```python
from build123d import *

# Parameters (mm, degrees)
F0_W      = 807.212
F0_H      = 403.86
F1_DEPTH  = 250.444
F2_R      = 60.325
F3_DEPTH  = 49.276
F4_T      = -25.4
F5_R      = 65.0773908114
F6_DEPTH  = 222.25
F7_R      = 62.8893110404
F8_DEPTH  = 222.25
F9_R      = 59.4615536077
F10_DEPTH = 222.25
F11_T     = -7.62


with BuildPart() as f1:
    # F0 (on Front) → F1 (new body)
    with BuildSketch(Plane.XZ):
        with Locations((41.8836543641, 201.93)):
            Rectangle(F0_W, F0_H)
    extrude(amount=F1_DEPTH)

    # F2 (on face) → F3 (join)
    with BuildSketch(Plane.XZ.offset(250.444)):
        with Locations((-263.2973456359, 309.245)):
            Circle(F2_R)
        with Locations((-263.2973456359, 106.045)):
            Circle(F2_R)
        with Locations((-60.0973456359, 309.245)):
            Circle(F2_R)
        with Locations((-60.0973456359, 106.045)):
            Circle(F2_R)
        with Locations((143.1026543641, 309.245)):
            Circle(F2_R)
        with Locations((143.1026543641, 106.045)):
            Circle(F2_R)
        with Locations((346.3026543641, 309.245)):
            Circle(F2_R)
        with Locations((346.3026543641, 106.045)):
            Circle(F2_R)
    extrude(amount=F3_DEPTH)

    # F4
    f4_openings = [f1.faces().sort_by_distance(p)[0] for p in [
        (41.883654, 0, 201.93),
    ]]
    offset(amount=F4_T, openings=f4_openings, kind=Kind.INTERSECTION)

    # F5 (on face) → F6 (join)
    with BuildSketch(Plane(origin=(0, -225.044, 0), x_dir=(-1, 0, 0), z_dir=(0, 1, 0))):
        with Locations((-246.4204579592, 209.5521092415)):
            Circle(F5_R)
    extrude(amount=F6_DEPTH)

    # F7 (on face) → F8 (join)
    with BuildSketch(Plane(origin=(0, -225.044, 0), x_dir=(-1, 0, 0), z_dir=(0, 1, 0))):
        with Locations((-39.1637831926, 205.74)):
            Circle(F7_R)
    extrude(amount=F8_DEPTH)

    # F9 (on face) → F10 (join)
    with BuildSketch(Plane(origin=(0, -225.044, 0), x_dir=(-1, 0, 0), z_dir=(0, 1, 0))):
        with Locations((166.5345877409, 205.74)):
            Circle(F9_R)
    extrude(amount=F10_DEPTH)

    # F11
    f11_openings = [f1.faces().sort_by_distance(p)[0] for p in [
        (246.420458, -2.794, 209.552109),
        (39.163783, -2.794, 205.74),
        (-166.534588, -2.794, 205.74),
    ]]
    offset(amount=F11_T, openings=f11_openings, kind=Kind.INTERSECTION)


solid = f1.part
```
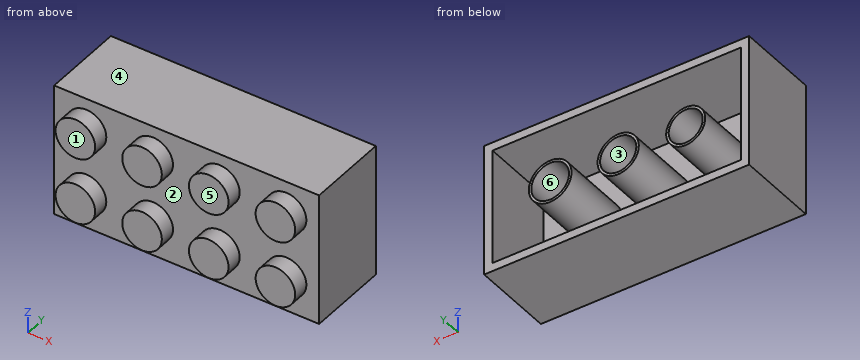
Could you check a few things on this model? Use its own coordinates, in mm. Face numbers are marked on the shaded views. A direction names the side the tool comes from. Give positions to 0.01 mm unless a question says otherwise; leave off trailing zeros. Write each loop counter-clockwise with the first axis right and the second up, starting at its lowest first coordinate (ties: lowest second). Pieces come first, ordered by that corner, then holes. Notation, with made-up numbers: (71.5, -5.5) -> (83.5, -5.5) arc R12 cw to (83.5, 16.5) -> close; hole circle Ø9 at (27.25, 61). An arc over 180 degrees is marked (long way). Write each question's results on one line, items separated by ' | '.
1. I want a section at A-A, the plane y = -57. Count the separate pieces of the cut face and the enclosed holes in it, then the cut area to 3 significant figures.
Check sheet entries:
separate pieces: 5 | enclosed holes: 5 | area: 43,800 mm²
2. On a 3-axis mill with a long thin cutter (end or side, diameter ignored), from which of +Z, -Z, +X, -X, +Y, -Y can I reach the whole of each face in a straight line? I mean the marked faces 5 and 6. Say none if no direction works.
Check sheet entries:
face 5: +Z, -Z, +X, -X, -Y | face 6: +Y
3. If we mould it in two halves opening along Z, with no side actions, what happens to the marked faces 1, 2, 3 and 4? For each: released by +Z, released by -Z, zero draft, split by the parting line, or undercut.
Check sheet entries:
face 1: zero draft | face 2: undercut | face 3: undercut | face 4: released by +Z
4. Will this pin go through, and if not, where does the flat tip stop? pin 1 Ø21 at (x, z) = (158.5, 308.5) entering from +Y.
Check sheet entries:
pin 1: stops at y = -274.32
5. I need wall thicknesses on L1, parallel to Z at x = -25.5, y = -225; L2, parallel to X at y = -101.5, z = 346; L3, parallel to Y at x = -300, z = 95. Which ranges of each line are inside material? Lowest first, please.
Check sheet entries:
L1: z = 0 to 7.62, 17.78 to 25.4, 378.46 to 386.08, 396.24 to 403.86 | L2: x = -361.72 to -354.1, -343.94 to -336.32, 420.09 to 427.71, 437.87 to 445.49 | L3: y = -299.72 to -292.1, -281.94 to -225.04
6. I want a section at B-B, the plane x = 217.5. Write out the boundary of the cut face in (y, z).
Check sheet entries:
outline: (-250.44, 0) -> (0, 0) -> (0, 25.4) -> (-225.04, 25.4) -> (-225.04, 151.25) -> (-2.79, 151.25) -> (-2.79, 159.9) -> (-232.66, 159.9) -> (-232.66, 17.78) -> (-7.62, 17.78) -> (-7.62, 7.62) -> (-242.82, 7.62) -> (-242.82, 396.24) -> (-7.62, 396.24) -> (-7.62, 386.08) -> (-232.66, 386.08) -> (-232.66, 259.2) -> (-2.79, 259.2) -> (-2.79, 267.85) -> (-225.04, 267.85) -> (-225.04, 378.46) -> (0, 378.46) -> (0, 403.86) -> (-250.44, 403.86) -> close
